```python
from build123d import *

# Parameters (mm, degrees)
SKETCH1_W                      = 44.45
SKETCH1_H                      = 38.1
SKETCH1_R                      = 1.1176
SKETCH1_R_2                    = 0.6858
SKETCH1_R_3                    = 1.27
BOSS_EXTRUDE1_DEPTH            = 1.5748
SKETCH2_R                      = 0.8001
SKETCH2_R_2                    = 0.381
SKETCH2_R_3                    = 1.4224
SWITCH_AND_R_A_CONNECTOR_DEPTH = 1.5748


with BuildPart() as part:
    # Sketch1 → Boss-Extrude1 (new body)
    with BuildSketch(Plane(origin=(0, 0, 0), x_dir=(1, 0, 0), z_dir=(0, 1, 0))):
        Rectangle(SKETCH1_W, SKETCH1_H)
        with Locations((-15.24, -12.065)):
            Circle(SKETCH1_R, mode=Mode.SUBTRACT)
        with Locations((1.651, -16.002)):
            Circle(SKETCH1_R_2, mode=Mode.SUBTRACT)
        with Locations((-7.112, -15.748)):
            Circle(SKETCH1_R_2, mode=Mode.SUBTRACT)
        with Locations((-11.43, -8.255)):
            Circle(SKETCH1_R_3, mode=Mode.SUBTRACT)
        with Locations((-11.43, -15.875)):
            Circle(SKETCH1_R_3, mode=Mode.SUBTRACT)
        with Locations((-19.05, -15.875)):
            Circle(SKETCH1_R_3, mode=Mode.SUBTRACT)
        with Locations((-19.05, -8.255)):
            Circle(SKETCH1_R_3, mode=Mode.SUBTRACT)
        with Locations((15.367, -12.065)):
            Circle(SKETCH1_R, mode=Mode.SUBTRACT)
        with Locations((19.177, -15.875)):
            Circle(SKETCH1_R_3, mode=Mode.SUBTRACT)
        with Locations((19.177, -8.255)):
            Circle(SKETCH1_R_3, mode=Mode.SUBTRACT)
        with Locations((11.557, -8.255)):
            Circle(SKETCH1_R_3, mode=Mode.SUBTRACT)
        with Locations((11.557, -15.875)):
            Circle(SKETCH1_R_3, mode=Mode.SUBTRACT)
        with Locations((1.143, -5.334)):
            Circle(SKETCH1_R, mode=Mode.SUBTRACT)
        with Locations((4.953, -9.144)):
            Circle(SKETCH1_R_3, mode=Mode.SUBTRACT)
        with Locations((4.953, -1.524)):
            Circle(SKETCH1_R_3, mode=Mode.SUBTRACT)
        with Locations((-2.667, -1.524)):
            Circle(SKETCH1_R_3, mode=Mode.SUBTRACT)
        with Locations((-2.667, -9.144)):
            Circle(SKETCH1_R_3, mode=Mode.SUBTRACT)
        with Locations((-2.64167216, -13.335)):
            Circle(SKETCH1_R_2, mode=Mode.SUBTRACT)
        with Locations((15.367, 1.905)):
            Circle(SKETCH1_R, mode=Mode.SUBTRACT)
        with Locations((11.557, -1.905)):
            Circle(SKETCH1_R_3, mode=Mode.SUBTRACT)
        with Locations((19.177, -1.905)):
            Circle(SKETCH1_R_3, mode=Mode.SUBTRACT)
        with Locations((19.177, 5.715)):
            Circle(SKETCH1_R_3, mode=Mode.SUBTRACT)
        with Locations((11.557, 5.715)):
            Circle(SKETCH1_R_3, mode=Mode.SUBTRACT)
        with Locations((6.12132784, -13.589)):
            Circle(SKETCH1_R_2, mode=Mode.SUBTRACT)
    extrude(amount=BOSS_EXTRUDE1_DEPTH)

    # Sketch2 → Switch and R A connector (cut)
    with BuildSketch(Plane(origin=(0, 1.5748, 0), x_dir=(1, 0, 0), z_dir=(0, 1, 0))):
        with Locations((0, 9.906)):
            Circle(SKETCH2_R)
        with Locations((-17.6022, 5.0546)):
            Circle(SKETCH2_R_2)
        with Locations((-17.6022, 2.5654)):
            Circle(SKETCH2_R_2)
        with Locations((-17.60295026, 0.083282904)):
            Circle(SKETCH2_R_2)
        with Locations((-15.0876, 5.0546)):
            Circle(SKETCH2_R_2)
        with Locations((-15.0876, 2.5654)):
            Circle(SKETCH2_R_2)
        with Locations((-15.0876, 0.0762)):
            Circle(SKETCH2_R_2)
        with Locations((-5.08, 10.541)):
            Circle(SKETCH2_R_3)
        with Locations((5.08, 10.541)):
            Circle(SKETCH2_R_3)
        with Locations((0, 15.621)):
            Circle(SKETCH2_R_3)
    extrude(amount=-SWITCH_AND_R_A_CONNECTOR_DEPTH, mode=Mode.SUBTRACT)


solid = part.part
```
Geometry: final body of the model. Coordinates: model frame, mm. Round coordinates to 2 decimals unless told otherwise and drop trailing zeros. Write each loop counter-clockwise with the first axis right and the second up, starting at its lowest first coordinate (ties: lowest second). Pieces come first, ordered by that corner, then holes.
Item 1: Pin query (flat end, axial travel): P1, Ø3.5, axis at x = 11.557, z = 8.255, coming from the -Y side. Return the tip coordinate at first contact, or that it passes through.
Item 2: Section query C-C (y = 1.05). Give the number of separate pieces and of enclosed holes in the cut face, plus the area to 3 significant figures.
Item 3: Material intervals for L1, parallel to Z at x = 5, y = 0.7; L2, parallel to X at y = 0.4, z = -5.5 (3 decimals); L3, parallel to X at y = 1.25, z = 13 (3 decimals), sorted ascending.
Item 4: Mould query, pull axis Z, two halves, no side actions, for faces 1 (the face through (0, 0, 0)), 2 (the face through (0, 1, 19.05)), 3 (the face through (-0.1, 0.8, -10.7)). Classes: +Z half, -Z half, draft (parallel to the pull), parting line (faces both ways), or undercut.
Item 5: Section query A-A (x = -5.08). Return loops of the section in (y, z).
Item 6: Section query B-B (x = -11.43). Return loops of the section in (y, z) (3 decimals), plus the area to 3 significant figures.
Completed:
1. P1: stops at y = 0
2. separate pieces: 1
2. enclosed holes: 34
2. area: 1,570 mm2
3. L1: z = -19.05 to -11.96, -9.12 to 0.25, 2.79 to 7.87, 10.41 to 19.05
3. L2: x = -22.225 to 10.305, 12.809 to 17.925, 20.429 to 22.225
3. L3: x = -22.225 to -15.852, -14.628 to -3.24, -2.043 to 5.77, 6.473 to 14.755, 15.979 to 22.225
4. face 1: draft
4. face 2: +Z half
4. face 3: undercut
5. outline: (0, -19.05) - (1.57, -19.05) - (1.57, -11.96) - (0, -11.96) - close; (0, -9.12) - (1.57, -9.12) - (1.57, 19.05) - (0, 19.05) - close
6. outline: (0, -19.05) - (1.575, -19.05) - (1.575, 6.985) - (0, 6.985) - close; (0, 9.525) - (1.575, 9.525) - (1.575, 14.605) - (0, 14.605) - close; (0, 17.145) - (1.575, 17.145) - (1.575, 19.05) - (0, 19.05) - close
6. area: 52.0 mm2
